Verification items for the finished model (mm, model axes). Face numbers are marked on the shaded views. A direction names the side the tool comes from. Round coordinates to 2 decimals unless told otherwise and drop trailing zeros. Write each loop counter-clockwise with the first axis right and the second up, starting at its lowest first coordinate (ties: lowest second). Pieces come first, ordered by that corner, then holes. Notation, with made-up numbers: M -31,-38 L 23,-38 A16 ccw 23,-26 Z; hole C 60.5,31.25 d8. An arc over 180 degrees is marked long. One line per item, written item: value. Start each with the question number.
Item 1: Thickness scan on probe 1 along Z at (x, y) = (0, -1.7); probe 2 along Z at (x, y) = (0, -1). Record the ranges inside material, lowest first. Write a range as from..to.
Item 2: Draft check along Z on the marked faces 3, 4 and 5. Enter one of: +Z half, -Z half, draft (parallel to the pull), parting line (faces both ways), or undercut.
Item 3: Gauge pin test, flat ends, axial feed: pin 1 (2 mm diameter, centred on x = 9, z = 8, fed in from +Y); pin 2 (1.5 mm diameter, centred on x = 1.5, y = -1.5, fed in from +Z). Record the tip position at first contact, or that the pin passes through.
Item 4: Section check A-A, the plane x = 0. State how many separate pieces and enclosed holes the cut face has, then the cut area to 3 significant figures.
Item 5: Section check C-C, the plane y = -0.95. Record the cut outline in (x, z), then the cut area to 3 significant figures.
Item 6: Section check D-D, the plane x = 9.5. Record the cut outline in (y, z), then the cut area to 3 significant figures.
Item 7: Tool access check on the marked faces 1 and 2. Record the directions out of +Z, -Z, +X, -X, +Y, -Y that give a thin tool (end or side, any length) a straight path to the whole face; none if there is none.
from build123d import *

# Parameters (mm, degrees)
SKETCH1_R                 = 15
SKETCH1_R_2               = 3
BOSS_EXTRUDE1_DEPTH       = 2.5
F_3_0MM_DOWEL_HOLE1_D     = 3
F_3_0MM_DOWEL_HOLE1_DEPTH = 5.001
CIRPATTERN1_COUNT         = 4
SKETCH6_R                 = 14
SKETCH6_R_2               = 7
CUT_EXTRUDE1_DEPTH        = 1


with BuildPart() as part:
    # Sketch1 → Boss-Extrude1 (new body, symmetric)
    with BuildSketch(Plane(origin=(0, 0, 0), x_dir=(1, 0, 0), z_dir=(0, 1, 0))):
        Circle(SKETCH1_R)
        Circle(SKETCH1_R_2, mode=Mode.SUBTRACT)
    extrude(amount=BOSS_EXTRUDE1_DEPTH, both=True)

    # Ø3.0mm Dowel Hole1
    with Locations(Plane(origin=(0, 2.5, 0), x_dir=(1, 0, 0), z_dir=(0, 1, 0))):
        with Locations((0, 10)):
            f_3_0mm_dowel_hole1 = Hole(F_3_0MM_DOWEL_HOLE1_D / 2, depth=F_3_0MM_DOWEL_HOLE1_DEPTH)

    # CirPattern1: Ø3.0mm Dowel Hole1 ×4 about axis
    cirpattern1_axis = Axis((0, 0, 0), (0, 1, 0))
    for i in range(1, CIRPATTERN1_COUNT):
        add(f_3_0mm_dowel_hole1.rotate(cirpattern1_axis, i * 360 / CIRPATTERN1_COUNT), mode=Mode.SUBTRACT)

    # Sketch6 → Cut-Extrude1 (cut)
    with BuildSketch(Plane(origin=(0, 2.5, 0), x_dir=(1, 0, 0), z_dir=(0, 1, 0))):
        Circle(SKETCH6_R)
        Circle(SKETCH6_R_2, mode=Mode.SUBTRACT)
    cut_extrude1 = extrude(amount=-CUT_EXTRUDE1_DEPTH, mode=Mode.SUBTRACT)

    # Mirror1: Cut-Extrude1 across plane
    add(cut_extrude1.mirror(Plane.ZX), mode=Mode.SUBTRACT)


solid = part.part
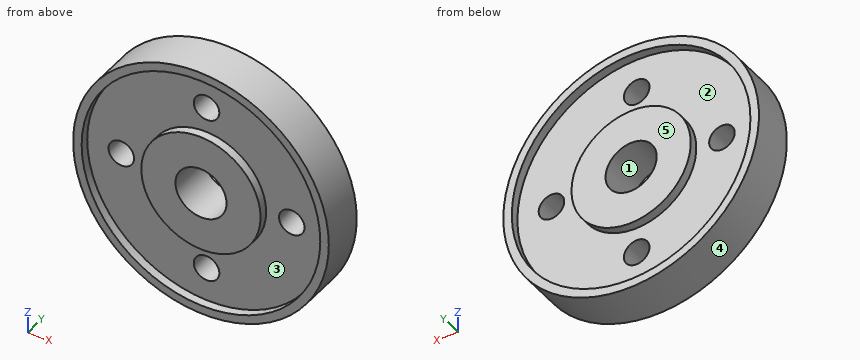
Response values:
1. probe 1: z = -15..-14, -7..-3, 3..7, 14..15
1. probe 2: z = -15..-11.5, -8.5..-3, 3..8.5, 11.5..15
2. face 3: undercut
2. face 4: parting line
2. face 5: draft
3. pin 1: stops at y = 1.5
3. pin 2: stops at z = 14.98
4. separate pieces: 4
4. enclosed holes: 0
4. area: 74.0 mm2
5. outline: C 0,0 d30; hole C -10,0 d3; hole C 0,0 d6; hole C 0,-10 d3; hole C 0,10 d3; hole C 10,0 d3
5. area: 650 mm2
6. outline: M -2.5,-11.61 L 2.5,-11.61 L 2.5,-10.28 L 1.5,-10.28 L 1.5,-1.41 L -1.5,-1.41 L -1.5,-10.28 L -2.5,-10.28 Z; M -2.5,10.28 L -1.5,10.28 L -1.5,1.41 L 1.5,1.41 L 1.5,10.28 L 2.5,10.28 L 2.5,11.61 L -2.5,11.61 Z
6. area: 66.5 mm2
7. face 1: +Y, -Y
7. face 2: +Y
